Verification items for the finished model (mm, model axes). A direction names the side the tool comes from. Coordinates: 2 decimals unless noted, no trailing zeros. Order: outer loops, then holes, each group sorted by start corner. A loop starts at its lowest first (then second) coordinate and runs counter-clockwise, first axis right, second up. Notation, with made-up numbers: (76, 28.5) -> (81, 28.5) arc R25 ccw to (81, 41.5) -> close; hole circle Ø2 at (7.5, 11). An arc over 180 degrees is marked (long way). Use CSV: the item, a comma, the result in double quotes. Start each with the question number.
1) Scan lines: line 1 along X through (y, z) = (-49, 58.5); line 2 along X through (y, z) = (-32.5, -32.5); line 3 along X through (y, z) = (-50.5, -11). Record each from-to range of solid material in increasing order.
2) Go/stop test with flat-tipped pins: pin 1 (1.1 mm diameter, centred on x = -11.5, y = -49, fed in from +Z); pin 2 (12 mm diameter, centred on x = -8.5, z = -16.5, fed in from -Y). Record where each tip stops, or that it passes through.
3) Sectioned sample at C-C on z = -15.5. Record the boundary of the cut face in (x, y), then the cut area to 3 significant figures.
4) Tool access check on faces 5 (the cylindrical face through (-8.667, -37.567, -38.081)), 6 (the cylindrical face through (23.64, -37.57, -78.34)). Record the directions out of +Z, -Z, +X, -X, +Y, -Y that give a thin tool (end or side, any length) a straight path to the whole face; none if there is none.
5) Release check for a two-part mould opening along X. For faces 1 (the cylindrical face through (-14.92, -37.567, -37.824)), 2 (the flat face through (25.4, -38, -1)), 3 (the flat face through (-25.4, -38, -54)), 4 (the flat face through (5, -76.2, -17)) record: released by +X, released by -X, zero draft, split by the parting line, or undercut.
6) Sectioned sample at B-B on x = 2. Record the boundary of the cut face in (y, z), then the cut area to 3 significant figures.
from build123d import *

# Parameters (mm, degrees)
F1_DEPTH = 76.2


# Not quite as in the source:
# - ends of sketch curves that miss each other by under 0.0002 mm in the source are joined


with BuildPart() as f1:
    # F0 (on Front) → F1 (new body)
    with BuildSketch(Plane.XZ):
        with BuildLine():
            Line((-25.4, -33.9672422), (-25.4, -74.1627422))
            ThreePointArc((-25.4, -74.1627422), (-23.6889178157, -78.2936600157), (-19.558, -80.0047422))
            Line((-19.558, -80.0047422), (19.558, -80.0047422))
            ThreePointArc((19.558, -80.0047422), (23.6889178157, -78.2936600157), (25.4, -74.1627422))
            Line((25.4, -74.1627422), (25.4, 74.1618532))
            ThreePointArc((25.4, 74.1618532), (23.6889178157, 78.2927710157), (19.558, 80.0038532))
            Line((19.558, 80.0038532), (18.3634634, 80.0038532))
            ThreePointArc((18.3634634, 80.0038532), (13.9275587532, 77.9297664461), (12.844644278, 73.1541629443))
            ThreePointArc((12.844644278, 73.1541629443), (12.9337447112, 72.6965968013), (12.9860822326, 72.2333837478))
            ThreePointArc((12.9860822326, 72.2333837478), (9.8726352632, 17.0060097148), (-7.2204417887, -35.601816093))
            ThreePointArc((-7.2204417887, -35.601816093), (-7.3997485398, -36.0211585586), (-7.5457824697, -36.4532160254))
            ThreePointArc((-7.5457824697, -36.4532160254), (-8.6899630694, -38.0977002575), (-10.5910126, -38.7297422))
            Line((-10.5910126, -38.7297422), (-12.7, -38.7297422))
            ThreePointArc((-12.7, -38.7297422), (-14.9450640303, -37.7998062303), (-15.875, -35.5547422))
            Line((-15.875, -35.5547422), (-15.875, -33.9672422))
            ThreePointArc((-15.875, -33.9672422), (-17.2699039546, -30.5996461546), (-20.6375, -29.2047422))
            ThreePointArc((-20.6375, -29.2047422), (-24.0050960454, -30.5996461546), (-25.4, -33.9672422))
        make_face()
    extrude(amount=F1_DEPTH)


solid = f1.part
Answers follow:
1,line 1,"x = 13.54 to 25.4"
1,line 2,"x = -25.17 to -16.11, -5.78 to 25.4"
1,line 3,"x = 2.65 to 25.4"
2,pin 1,"stops at z = -38.73"
2,pin 2,"passes through"
3,outline,"(1.1, -76.2) -> (25.4, -76.2) -> (25.4, 0) -> (1.1, 0) -> close"
3,area,"1,850 mm²"
4,face 5,"+Z, +Y, -Y"
4,face 6,"-Z, +X, +Y, -Y"
5,face 1,"undercut"
5,face 2,"released by +X"
5,face 3,"released by -X"
5,face 4,"zero draft"
6,outline,"(-76.2, -80) -> (0, -80) -> (0, -12.92) -> (-76.2, -12.92) -> close"
6,area,"5,110 mm²"
